```python
from build123d import *

# Parameters (mm, degrees)
SKETCH_1_W                 = 76
SKETCH_1_H                 = 46
EXTRUDE_1_DEPTH            = 15
CUT_EXTRUDE_1_REACH        = 92.094
SKETCH_2_R                 = 14
CUT_EXTRUDE_3_DEPTH        = 91.094394942
CUT_EXTRUDE_4_REACH        = 92.094
CUT_EXTRUDE_4_END_RADIUS   = 14
HOLE_WIZARD_M41_AT_2_COUNT = 2
HOLE_WIZARD_M41_AT_2_PITCH = 55
HOLE_WIZARD_M42_AT_2_COUNT = 2
HOLE_WIZARD_M42_AT_2_PITCH = 55
SKETCH_15_W                = 4
SKETCH_15_H                = 6.19823693
SKETCH_15_H_2              = 5.19823693
CUT_EXTRUDE_START          = -4
CUT_EXTRUDE_5_DEPTH        = 4


# Read off the part's stored shape, not the designer's step: Отверстие обработанное метчиком M31, Отверстие обработанное метчиком M32
with BuildPart() as part:
    # Эскиз1 → Бобышка-Вытянуть1 (new body)
    with BuildSketch(Plane.XY):
        with Locations((38, 23)):
            Rectangle(SKETCH_1_W, SKETCH_1_H)
    extrude(amount=EXTRUDE_1_DEPTH)

    # Эскиз2 → Вырез-Вытянуть1 (cut, up to next)
    with BuildSketch(Plane.XY.offset(15), mode=Mode.PRIVATE) as cut_extrude_1_sk1:
        with Locations((35, 23)):
            Circle(SKETCH_2_R)
    cut_extrude_1_tool1 = extrude(cut_extrude_1_sk1.sketch, amount=-CUT_EXTRUDE_1_REACH, mode=Mode.PRIVATE) & part.part
    add(cut_extrude_1_tool1.solids().sort_by_distance((35, 23, 15))[0], mode=Mode.SUBTRACT)

    # Эскиз3 → Вырез-Вытянуть3 (cut, through all)
    with BuildSketch(Plane.XY.offset(15)):
        Polygon((17, 10), (4, 10), (4, 17), (12, 17), (12, 36), (0, 36), (0, 0), (17, 0), align=None)
        Polygon((53, 10), (53, 0), (76, 0), (76, 36), (58, 36), (58, 17), (72, 17), (72, 10), align=None)
    extrude(amount=-CUT_EXTRUDE_3_DEPTH, mode=Mode.SUBTRACT)

    # Вырез-Вытянуть4: up to this cylinder (the profile starts outside it)
    cut_extrude_4_end = Plane(origin=(35, 23, 1.635023), z_dir=(0, 0, 1)) * Cylinder(CUT_EXTRUDE_4_END_RADIUS, 213.188, mode=Mode.PRIVATE)
    # Эскиз4 → Вырез-Вытянуть4 (cut, up to the surface)
    with BuildSketch(Plane(origin=(0, 46, 0), x_dir=(1, 0, 0), z_dir=(0, 1, 0)), mode=Mode.PRIVATE) as cut_extrude_4_sk1:
        with BuildLine():
            Line((42.483314774, 0), (27.516685226, 0))
            ThreePointArc((27.516685226, 0), (35, -4), (42.483314774, 0))
        make_face()
    cut_extrude_4_tool1 = extrude(cut_extrude_4_sk1.sketch, amount=-CUT_EXTRUDE_4_REACH, mode=Mode.PRIVATE) - cut_extrude_4_end
    add(cut_extrude_4_tool1.solids().sort_by_distance((35, 46, 1.635023))[0], mode=Mode.SUBTRACT)

    # Эскиз5 → Вырез-Повернуть1 (revolve, cut)
    with BuildSketch(Plane(origin=(0, 23, 0), x_dir=(-1, 0, 0), z_dir=(0, 1, 0)), mode=Mode.PRIVATE) as cut_revolve_1_sk:
        Polygon((15, 15), (-13, 15), (-13, 12), (-17, 12), (-17, 8), (15, 8), align=None)
        Polygon((-21.564689936, 15), (-20, 15), (-21.564689936, 6.126202411), align=None)
    revolve(cut_revolve_1_sk.sketch.rotate(Axis((35, 23, 0), (0, 0, 1)), 180), axis=Axis((35, 23, 0), (0, 0, 1)), mode=Mode.SUBTRACT)

    # Эскиз6 → Отверстие обработанное метчиком M41 (revolve, cut)
    with BuildSketch(Plane(origin=(9, 46, 5), x_dir=(0, 0, 1), z_dir=(1, 0, 0))):
        Polygon((0, 0), (0, 10), (2.175, 10), (1.65, 9.475), (1.65, 0.367608958), (2.175, 0), align=None)
    hole_wizard_m41 = revolve(axis=Axis((9, 52.35, 5), (0, -1, 0)), mode=Mode.SUBTRACT)

    # Отверстие обработанное метчиком M41 at 2: Отверстие обработанное метчиком M41 ×2
    with Locations(*[(i * HOLE_WIZARD_M41_AT_2_PITCH, 0, 0) for i in range(1, HOLE_WIZARD_M41_AT_2_COUNT)]):
        add(hole_wizard_m41, mode=Mode.SUBTRACT)

    # Эскиз8 → Отверстие обработанное метчиком M42 (revolve, cut)
    with BuildSketch(Plane(origin=(64, 10, 5), x_dir=(0, 0, -1), z_dir=(1, 0, 0))):
        Polygon((0, 0), (0, 7), (2.175, 7), (1.65, 6.475), (1.65, 0.367608958), (2.175, 0), align=None)
    hole_wizard_m42 = revolve(axis=Axis((64, 3.65, 5), (0, 1, 0)), mode=Mode.SUBTRACT)

    # Отверстие обработанное метчиком M42 at 2: Отверстие обработанное метчиком M42 ×2
    with Locations(*[(-i * HOLE_WIZARD_M42_AT_2_PITCH, 0, 0) for i in range(1, HOLE_WIZARD_M42_AT_2_COUNT)]):
        add(hole_wizard_m42, mode=Mode.SUBTRACT)

    # Отверстие обработанное метчиком M31 outline → Отверстие обработанное метчиком M31 (revolve, cut)
    with BuildSketch(Plane(origin=(0, 41, 5), x_dir=(0, 1, 0), z_dir=(0, 0, -1))):
        Polygon((1.25, 0.315093392), (1.25, 7.923293242), (0, 7.923293242), (0, 0), (1.7, 0), align=None)
    revolve(axis=Axis((0, 41, 5), (1, 0, 0)), mode=Mode.SUBTRACT)

    # Отверстие обработанное метчиком M32 outline → Отверстие обработанное метчиком M32 (revolve, cut)
    with BuildSketch(Plane(origin=(0, 41, 5), x_dir=(0, 1, 0), z_dir=(0, 0, -1))):
        Polygon((0, 65.076706758), (1.25, 65.076706758), (1.25, 75.684906608), (1.7, 76), (0, 76), align=None)
    revolve(axis=Axis((0, 41, 5), (1, 0, 0)), mode=Mode.SUBTRACT)

    # Эскиз15 → Вырез-Повернуть2 (revolve, cut)
    with BuildSketch(Plane(origin=(0, 0, 5), x_dir=(-1, 0, 0), z_dir=(0, 0, -1)), mode=Mode.PRIVATE) as cut_revolve_2_sk:
        with Locations((-2, 33.900881535)):
            Rectangle(SKETCH_15_W, SKETCH_15_H)
        with Locations((-74, 33.400881535)):
            Rectangle(SKETCH_15_W, SKETCH_15_H_2)
    revolve(cut_revolve_2_sk.sketch.rotate(Axis((8.006810355, 41, 5), (-1, 0, 0)), 270), axis=Axis((8.006810355, 41, 5), (-1, 0, 0)), mode=Mode.SUBTRACT)

    # Эскиз16 → Вырез-Вытянуть5 (cut)
    with BuildSketch(Plane.XY.offset(15).offset(CUT_EXTRUDE_START)):
        with BuildLine():
            Line((18, 9.035759956), (18, 36.964240044))
            ThreePointArc((18, 36.964240044), (13, 23), (18, 9.035759956))
        make_face()
        with BuildLine():
            ThreePointArc((57, 23), (55.712315177, 30.416198487), (52, 36.964240044))
            Line((52, 36.964240044), (52, 9.035759956))
            ThreePointArc((52, 9.035759956), (55.712315177, 15.583801513), (57, 23))
        make_face()
    extrude(amount=CUT_EXTRUDE_5_DEPTH, mode=Mode.SUBTRACT)


solid = part.part
```
CAD build for the part. Positions are in the model's coordinates, mm. A direction names the side the tool comes from. Round coordinates to 2 decimals unless told otherwise and drop trailing zeros. Loops run counter-clockwise (first coordinate to the right, second up) from the corner with the lowest first, then second, coordinate; pieces in that order, holes last. Notation, with made-up numbers: (-7.75, 59.25) - (14.25, 59.25) arc R25 ccw to (14.25, 89.25) - close; hole circle Ø1 at (16.5, 75). An arc over 180 degrees is marked (long way). Return JSON: item names as keys, results as strings. Group by question number.
Q1. Flat gauge pins, fed straight in: pin 1 Ø1 at (y, z) = (9, 3) entering from -X; pin 2 Ø9 at (x, z) = (65, 2.5) entering from -Y; pin 3 Ø4.5 at (y, z) = (28.5, 12) entering from -X. Where does each tip first touch, or does it go through?
Q2. Band-saw the part on B-B on y = 23. Give the cut face in (x, z).
Q3. Drill centre lines: line 1 along Y through (x, z) = (68, 5); line 2 along X through (y, z) = (43.25, 5); line 3 along Z through (x, y) = (9, 42). Where is each one in solid material? Low to high. Write a range as [from, to].
Q4. Band-saw the part on A-A on x = 71. Give the cut face in (y, z), plus the area to 3 significant figures.
Q5. Band-saw the part on D-D on z = 13. Give the cut face in (x, y), plus the area to 3 significant figures.
Q6. Tool access for faces 5 (the face through (17, 5, 4)), 6 (the face through (72, 45, 1)), 7 (the face through (70.46, 40.01, 4.24)): list every direction of +Z, -Z, +X, -X, +Y, -Y with a clear straight run to the whole face (end or side of a thin tool).
Q7. Two-plate mould, pull along X, no slides. Class faces 1 (the face through (76, 41, 3)), 2 (the face through (2, 41, 1)), 3 (the face through (48.4, 27.22, 9.6)), 4 (the face through (65.6, 13.4, 5.4)): +X half, -X half, draft (parallel to the pull), parting line (faces both ways), or undercut.
Q8. Band-saw the part on C-C on x = 35. Give the cut face in (y, z).
Solutions:
{
 "1": {"pin 1": "stops at x = 17", "pin 2": "stops at y = 10", "pin 3": "stops at x = 17.34"},
 "2": {"outline": "(12, 0) - (21, 0) - (21, 9.33) - (20, 15) - (18, 15) - (18, 11) - (17, 11) - (17, 8) - (12, 8) - close; (49, 0) - (58, 0) - (58, 8) - (53, 8) - (53, 11) - (52, 11) - (52, 15) - (50, 15) - (49, 9.33) - close"},
 "3": {"line 1": "y = [10, 17], [36, 39.75], [42.25, 46]", "line 2": "x = [0, 7.35], [10.65, 62.35], [65.65, 76]", "line 3": "z = [0, 3.35], [6.65, 8]"},
 "4": {"outline": "(10, 0) - (17, 0) - (17, 8) - (10, 8) - close; (36, 0) - (46, 0) - (46, 8) - (36, 8) - close; hole circle Ø2.5 at (41, 5)", "area": "131 mm^2"},
 "5": {"outline": "(18, 9.04) arc R22 ccw to (52, 9.04) - (52, 36.96) arc R22 ccw to (18, 36.96) - close; hole circle Ø29.29 at (35, 23)", "area": "656 mm^2"},
 "6": {"face 5": "+Z, -Z, -X, -Y", "face 6": "-Z, +X, +Y", "face 7": "+X"},
 "7": {"face 1": "+X half", "face 2": "draft", "face 3": "undercut", "face 4": "undercut"},
 "8": {"outline": "(0, 0) - (9, 0) - (9, 9.33) - (8, 15) - (1, 15) - (1, 12) - (5, 12) - (5, 8) - (0, 8) - close; (37, 4) - (46, 4) - (46, 8) - (41, 8) - (41, 12) - (45, 12) - (45, 15) - (38, 15) - (37, 9.33) - close"}
}
